Autodesk Inventor part; units mm, degrees
ref_plane "YZ Plane" through (0, 0, 0) normal (1, 0, 0) x (0, 1, 0)
ref_plane "XZ Plane" through (0, 0, 0) normal (0, 1, 0) x (-1, 0, 0)
ref_plane "XY Plane" through (0, 0, 0) normal (0, 0, 1) x (1, 0, 0)
sketch "Skizze1" plane through (0, 0, 0) normal (1, 0, 0) x (0, 1, 0)
  line L0 (0, 0) -> (144, 0)
  line L1 (144, 0) -> (144, -68)
  line L2 (144, -68) -> (0, -68)
  line L3 (0, -68) -> (0, 0)
  dimension "d0" = 144
  dimension "d1" = 68
extrude "Extrusion1" add sketch "Skizze1" along normal blind 16
sketch "Skizze2" plane through (0, 0, 0) normal (0, 0, 1) x (1, 0, 0)
  line L0 (0, 0) -> (0, 144) construction
  line L1 (0, 72) -> (16, 72) construction
  line L2 (16, 144) -> (16, 0) construction
  line L3 (0, 144) -> (16, 144) construction
  line L4 (8, 144) -> (8, 0) construction
  line L5 (0, 144) -> (16, 144) construction
  line L6 (0, 0) -> (16, 0) construction
  line L7 (0, 144) -> (16, 144) construction
  line L8 (16, 144) -> (16, 0) construction
  line L9 (16, 0) -> (0, 0) construction
  line L10 (0, 0) -> (0, 144) construction
  line L11 (0, 112) -> (16, 112) construction
  line L12 (0, 32) -> (16, 32) construction
  point P0 (8, 112)
  point P1 (8, 72)
  point P2 (8, 32)
  dimension "d4" = 40
  dimension "d5" = 40
hole "Bohrung1" at (8, 112, 0) at (8, 32, 0) direction (0, 0, -1) diameter 2.5 depth 30 tip angle 118
sketch "Skizze3" plane through (0, 144, 0) normal (0, 1, 0) x (1, 0, 0)
  line L0 (0, 0) -> (16, 0)
  line L1 (16, 0) -> (16, 68)
  line L2 (16, 68) -> (0, 68)
  line L3 (0, 68) -> (0, 0)
  line L4 (8, 0) -> (8, 68) construction
  line L5 (0, 68) -> (16, 68) construction
  line L6 (16, 0) -> (16, 68) construction
  line L7 (16, 34) -> (0, 34) construction
  line L8 (0, 68) -> (0, 0) construction
  line L9 (0, 14) -> (16, 14) construction
  line L10 (0, 54) -> (16, 54) construction
  point P0 (8, 14)
  point P1 (8, 54)
  dimension "d13" = 14
  dimension "d22" = 14
hole "Bohrung2" at (8, 144, -14) at (8, 144, -54) direction (0, -1, 0) diameter 2.5 depth 25 tip angle 118
sketch "Skizze4" plane through (0, 0, -68) normal (0, 0, -1) x (-1, 0, 0)
  line L0 (0, 0) -> (-16, 0) construction
  line L1 (-16, 0) -> (-16, 144) construction
  line L2 (-16, 144) -> (0, 144) construction
  line L3 (0, 144) -> (0, 0) construction
  line L4 (-8, 0) -> (-8, 144) construction
  line L5 (-16, 144) -> (-16, 0) construction
  line L6 (-16, 72) -> (0, 72) construction
  point P0 (-8, 112)
  point P1 (-8, 32)
  dimension "d53" = 72
  dimension "d54" = 40
  dimension "d55" = 40
hole "Bohrung3" at (8, 112, -68) at (8, 32, -68) direction (0, 0, 1) diameter 2.5 depth 30 tip angle 118
sketch "Skizze5" plane through (16, 0, 0) normal (1, 0, 0) x (0, 0, -1)
  line L0 (68, 144) -> (0, 144) construction
  line L1 (0, 144) -> (0, 0) construction
  line L2 (0, 0) -> (68, 0) construction
  line L3 (68, 0) -> (68, 144) construction
  line L4 (0, 144) -> (0, 0) construction
  line L5 (0, 72) -> (68, 72) construction
  circle A0 centre (34, 72) radius 4 construction
  line L6 (20, 119) -> (20, 39) construction
  point P0 (20, 79)
  dimension "d41" = 8
  dimension "d42" = 7
  dimension "d43" = 40
  dimension "d44" = 40
  dimension "d45" = 20
hole "Bohrung4" at (16, 39, -20) at (16, 79, -20) at (16, 119, -20) direction (-1, 0, 0) diameter 4 end through all countersink diameter 8 countersink angle 90
hole "Bohrung5" at (16, 72, -34) direction (-1, 0, 0) diameter 10 end through all
sketch "Skizze6" plane through (0, 0, 0) normal (0, 0, 1) x (1, 0, 0)
  circle A0 centre (8, 112) radius 1.25
  circle A1 centre (8, 32) radius 1.25
  line L0 (0, 0) -> (0, 144)
  line L1 (0, 0) -> (16, 0)
  line L2 (16, 144) -> (16, 0)
  line L3 (0, 144) -> (16, 144)
  point P0 (8, 72)
  dimension "d56" = 40
hole "Bohrung6" at (8, 72, 0) direction (0, 0, -1) diameter 2.5 depth 25 tip angle 118
sketch "Skizze7" plane through (0, 0, -68) normal (0, 0, -1) x (-1, 0, 0)
  circle A0 centre (-8, 72) radius 1.25
  point P0 (0, 0)
hole "Bohrung7" at (8, 72, -68) direction (0, 0, 1) diameter 2.5 depth 25 tip angle 118
equation "\"d39\" = Stärke"
equation "\"d51\" = Stärke"
equation "\"Biegeradius\" = Stärke"
equation "\"BreiteBiegungsfreistellung\" = Stärke"
equation "\"TiefeBiegungsfreistellung\" = 0.5 * Stärke"
equation "\"GrößeEckenfreistellung\" = 4 * Stärke"
equation "\"MinimalRest\" = 2 * Stärke"
equation "\"Übergangsradius\" = Biegeradius"
equation "\"JacobiRadiusGröße\" = Biegeradius"
equation "\"Abstandsgröße\" = Stärke"
properties part number "licht_150_side_right" material "Spanplatte"
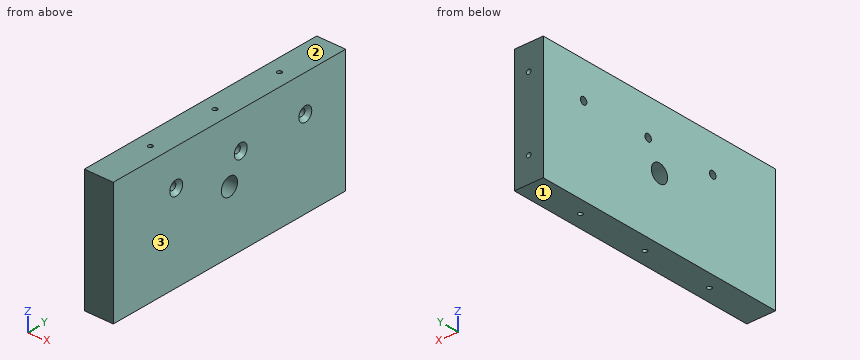
The listing builds one solid part. Answer for the finished solid, in the listing's coordinates (mm). Face numbers are marked on the shaded views. Round coordinates to 2 decimals unless told otherwise and drop trailing zeros. Order: outer loops, then holes, each group sorted by start corner. A loop starts at its lowest first (then second) coordinate and runs counter-clockwise, first axis right, second up. Notation, with made-up numbers: (16.5, 40.25) -> (27.5, 40.25) arc R18 ccw to (27.5, 57.25) -> close; hole circle Ø3 at (-29, 2.5). An arc over 180 degrees is marked (long way). One line per item, written item: value.
Item 1: For a pull along Z with two mould halves and no side action, classify the marked faces 1, 2 and 3 as released by +Z, released by -Z, zero draft, split by the parting line, or undercut.
Taken from the geometry:
face 1: released by -Z
face 2: released by +Z
face 3: zero draft
Item 2: Given P1, Ø2, axis at x = 8, z = -54, coming from the +Y side; P2, Ø1.5, axis at x = 8, y = 72, coming from the +Z side; P3, Ø2, axis at x = 8, y = 112, coming from the +Z side, each flat-ended and moving along its own axis, determine where each tip first touches the part or whether it passes through.
Taken from the geometry:
P1: stops at y = 118.85
P2: stops at z = -25.3
P3: stops at z = -30.15
Item 3: Find section B-B, the plane z = -34. Give the vertices of the cut face in (x, y).
Taken from the geometry:
outline: (0, 0) -> (16, 0) -> (16, 67) -> (0, 67) -> close; (0, 77) -> (16, 77) -> (16, 144) -> (0, 144) -> close
Item 4: Find section A-A, the plane z = -20. Give the vertices of the cut face in (x, y).
Taken from the geometry:
outline: (0, 0) -> (16, 0) -> (16, 35) -> (14, 37) -> (0, 37) -> close; (0, 41) -> (14, 41) -> (16, 43) -> (16, 75) -> (14, 77) -> (0, 77) -> close; (0, 81) -> (14, 81) -> (16, 83) -> (16, 115) -> (14, 117) -> (0, 117) -> close; (0, 121) -> (14, 121) -> (16, 123) -> (16, 144) -> (0, 144) -> close; hole circle Ø2.5 at (8, 32); hole circle Ø2.5 at (8, 72); hole circle Ø2.5 at (8, 112)
Item 5: Find section C-C, the plane y = 79. Give the vertices of the cut face in (x, z), then the cut area to 3 significant figures.
Taken from the geometry:
outline: (0, -68) -> (16, -68) -> (16, -24) -> (14, -22) -> (0, -22) -> close; (0, -18) -> (14, -18) -> (16, -16) -> (16, 0) -> (0, 0) -> close
area: 1,020 mm2
Item 6: Straight lines are drawn through the part: L1, parallel to Y at x = 8, z = -51.5; L2, parallel to Z at x = 8, y = 134.25; L3, parallel to Y at x = 10.5, z = -20. For each, find the intervals that lie inside material, in ascending order.
Taken from the geometry:
L1: y = 0 to 30.75, 33.25 to 70.75, 73.25 to 110.75, 113.25 to 144
L2: z = -68 to -55.25, -52.75 to -15.25, -12.75 to 0
L3: y = 0 to 37, 41 to 77, 81 to 117, 121 to 144
